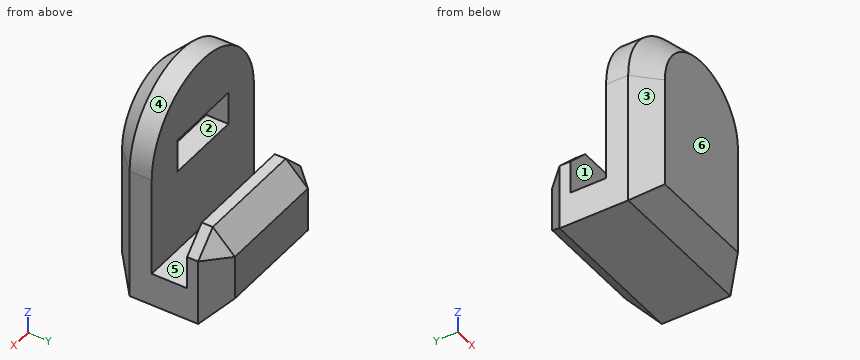
```python
from build123d import *

# Parameters (mm, degrees)
PAD_DEPTH            = 2
SKETCH001_W          = 3.5
SKETCH001_H          = 1.5
POCKET_DEPTH         = 1
SKETCH002_W          = 7
SKETCH002_H          = 1.5
PAD001_DEPTH         = 1.6
SKETCH003_W          = 7
SKETCH003_H          = 4
PAD002_DEPTH         = 1.5
CHAMFER_SIZE         = 1
CHAMFER001_SIZE      = 1
BODY_PLACEMENT_ANGLE = 90


with BuildPart() as part:
    # Sketch (on XY_Plane of Origin) → Pad (new body)
    with BuildSketch(Plane.XY):
        with BuildLine():
            Line((-3.5, -1.5), (-3.5, 4.5))
            ThreePointArc((3.5, 4.5), (0, 8), (-3.5, 4.5))
            Line((3.5, 4.5), (3.5, -1.5))
            Line((3.5, -1.5), (-3.5, -1.5))
        make_face()
    extrude(amount=PAD_DEPTH)

    # Sketch001 (on Face5 of Pad) → Pocket (cut)
    with BuildSketch(Plane(origin=(0, 0, 0), x_dir=(1, 0, 0), z_dir=(0, 0, -1))):
        with Locations((0, -4.5)):
            Rectangle(SKETCH001_W, SKETCH001_H)
    extrude(amount=-POCKET_DEPTH, mode=Mode.SUBTRACT)

    # Sketch002 (on Face4 of Pocket) → Pad001 (join)
    with BuildSketch(Plane(origin=(0, 0, 0), x_dir=(1, 0, 0), z_dir=(0, 0, -1))):
        with Locations((0, 0.75)):
            Rectangle(SKETCH002_W, SKETCH002_H)
    extrude(amount=PAD001_DEPTH)

    # Sketch003 (on Face10 of Pad001) → Pad002 (join)
    with BuildSketch(Plane(origin=(0, 0, -1.6), x_dir=(1, 0, 0), z_dir=(0, 0, -1))):
        with Locations((0, -0.5)):
            Rectangle(SKETCH003_W, SKETCH003_H)
    extrude(amount=PAD002_DEPTH)

    # Chamfer
    chamfer_edges = [part.edges().sort_by_distance(p)[0] for p in [
        (0, -1.5, -3.1),
        (-3.5, 0.5, -3.1),
        (3.5, 0.5, -3.1),
        (0, 2.5, -3.1),
        (-3.5, 2.5, -2.35),
        (3.5, 2.5, -2.35),
    ]]
    chamfer(chamfer_edges, length=CHAMFER_SIZE)

    # Chamfer001
    chamfer001_edges = [part.edges().sort_by_distance(p)[0] for p in [
        (0, 8, 2),
        (0, -1.5, 2),
    ]]
    chamfer(chamfer001_edges, length=CHAMFER001_SIZE)


with BuildPart() as part_1:
    # Body placement: moved
    add(part.part.rotate(Axis((0, 0, 0), (1, 0, 0)), BODY_PLACEMENT_ANGLE))


solid = part_1.part
```
Check sheet for the modelled part. Datum: model origin and axes. Units: mm. Face numbers are marked on the shaded views. A direction names the side the tool comes from. Give positions to 0.01 mm unless a question says otherwise; leave off trailing zeros. Write each loop counter-clockwise with the first axis right and the second up, starting at its lowest first coordinate (ties: lowest second). Pieces come first, ordered by that corner, then holes.
Item 1: Cross-section at B-B (z = 4). Enter the section's corners in (x, y), and give its area (3 significant figures).
Item 2: Scan lines: L1, parallel to Y at x = 0.25, z = 0.5; L2, parallel to Y at x = -1.25, z = 4.75; L3, parallel to Z at x = -3, y = 0.1. Record each from-to range of solid material in increasing order.
Item 3: Gauge pin test, flat ends, axial feed: pin 1 (2 mm diameter, centred on x = 0, z = 5, fed in from +Y); pin 2 (0.8 mm diameter, centred on x = -1.5, y = 1, fed in from +Z). Record the tip position at first contact, or that the pin passes through.
Item 4: Access from +Z, -Z, +X, -X, +Y, -Y to the whole of each face (thin tool, end or side, straight path). Record for the marked faces 1, 2 and 3.
Item 5: Cross-section at A-A (x = 0). Enter the section's corners in (y, z), and give its area (3 significant figures).
Item 6: Cross-section at D-D (y = 1.9). Enter the section's corners in (x, z).
Item 7: Cross-section at C-C (y = 2.55). Enter the section's corners in (x, z), and give its area (3 significant figures).
Item 8: Draft check along Y on the marked faces 4, 5 and 6. Enter one of: released by +Y, released by -Y, zero draft, split by the parting line, or undercut.
Report:
1. outline: (-3.5, -1) - (-2.5, -2) - (2.5, -2) - (3.5, -1) - (3.5, 0) - (1.75, 0) - (1.75, -1) - (-1.75, -1) - (-1.75, 0) - (-3.5, 0) - close
1. area: 9.50 mm2
2. L1: y = -2 to 0, 1.6 to 3.1
2. L2: y = -2 to -1
2. L3: z = -1.5 to 0
3. pin 1: stops at y = 0
3. pin 2: stops at z = 0
4. face 1: +Z, +X, -X
4. face 2: +Y
4. face 3: +Z, -Z, -X, -Y
5. outline: (-2, -0.5) - (-1, -1.5) - (2.1, -1.5) - (3.1, -0.5) - (3.1, 1.5) - (2.1, 2.5) - (1.6, 2.5) - (1.6, 0) - (0, 0) - (0, 3.75) - (-1, 3.75) - (-1, 5.25) - (0, 5.25) - (0, 8) - (-1, 8) - (-2, 7) - close
5. area: 23.9 mm2
6. outline: (-3.5, -1.5) - (3.5, -1.5) - (3.5, 1.5) - (2.5, 2.5) - (-2.5, 2.5) - (-3.5, 1.5) - close
7. outline: (-3.05, -1.05) - (3.05, -1.05) - (3.05, 1.5) - (2.5, 2.05) - (-2.5, 2.05) - (-3.05, 1.5) - close
7. area: 18.6 mm2
8. face 4: zero draft
8. face 5: undercut
8. face 6: released by -Y
